Verification items for the finished model (mm, model axes). Round coordinates to 2 decimals unless told otherwise and drop trailing zeros. Order: outer loops, then holes, each group sorted by start corner. A loop starts at its lowest first (then second) coordinate and runs counter-clockwise, first axis right, second up. Notation, with made-up numbers: M 81,-21.75 L 129,-21.75 A21 cw 129,-7.75 Z; hole C 72.25,70.25 d9. An arc over 180 degrees is marked long. Use CSV: the item, a comma, the result in double quotes. Start each with the question number.
Q1. Gauge pin test, flat ends, axial feed: pin 1 Ø18 at (x, y) = (-11, 3.5) entering from +Z; pin 2 Ø22 at (x, z) = (-11, -820) entering from -Y (3 decimals); pin 3 Ø2 at (x, z) = (-13.5, -747.5) entering from +Y (3 decimals). Record the tip position at first contact, or that the pin passes through.
Q2. Sectioned sample at A-A (z = -1361.5). Enter the section's corners in (x, y) (3 decimals).
Q3. Scan lines: line 1 (Y direction, x = 10.5, z = -1140) (3 decimals); line 2 (Z direction, x = 0.5, y = 33). Record each from-to range of solid material in increasing order.
Q4. Sectioned sample at B-B (y = -189). Enter the section's corners in (x, z), and give its area (3 significant figures).
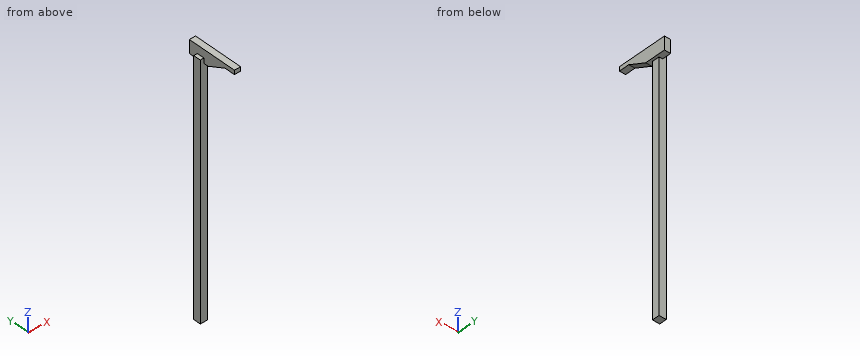
```python
from build123d import *

# Parameters (mm, degrees)
F0_W     = 44.45
F0_H     = 44.45
F1_DEPTH = 1524
F3_DEPTH = 38.1


with BuildPart() as f1:
    # F0 (on Top) → F1 (new body)
    with BuildSketch(Plane.XY):
        Rectangle(F0_W, F0_H)
    extrude(amount=-F1_DEPTH)

    # F2 (on Right) → F3 (join)
    with BuildSketch(Plane.YZ):
        Polygon((76.361727, -31.198649), (76.361727, 49.559367), (-228.438273, 49.559367), (-228.438273, 24.159367), (-164.938273, 24.159367), (-50.638273, -31.198649), align=None)
    extrude(amount=F3_DEPTH)


solid = f1.part
```
Verdict:
1,pin 1,"stops at z = 0"
1,pin 2,"stops at y = -22.225"
1,pin 3,"stops at y = 22.225"
2,outline,"M -22.225,-22.225 L 22.225,-22.225 L 22.225,22.225 L -22.225,22.225 Z"
3,line 1,"y = -22.225 to 22.225"
3,line 2,"z = -31.2 to 49.56"
4,outline,"M 0,24.16 L 38.1,24.16 L 38.1,49.56 L 0,49.56 Z"
4,area,"968 mm²"
